The model under review builds one solid part; all positions refer to its coordinate system, in mm. Give positions to 0.01 mm unless a question says otherwise; leave off trailing zeros. Loops run counter-clockwise (first coordinate to the right, second up) from the corner with the lowest first, then second, coordinate; pieces in that order, holes last. Notation, with made-up numbers: M -11.75,15.5 L 7.25,15.5 A16 cw 7.25,46.5 Z; hole C 1,66 d11. An arc over 180 degrees is marked long. Write item = value, one per line. Start each with the question number.
1. We need section A-A on x = 25.5. Give the boundary of the cut face in (y, z).
2. For pin 1 (7 mm diameter, centred on x = 25.5, z = 2, fed in from -Y); pin 2 (1 mm diameter, centred on y = 2, z = 6.5, fed in from -X), all flat-tipped, find the tip position at first contact; note any pin that passes through.
3. We need section B-B on y = 1.35. Give the boundary of the cut face in (x, z) (3 decimals).
4. We need section C-C on z = 7. Give the boundary of the cut face in (x, y).
5. Wall thickness on line 1 along Z through (x, y) = (19, 1.9); line 2 along X through (y, z) = (0.9, 1.5); line 3 along X through (y, z) = (1.9, 0.75): over which ranges is each line inside the solid? List them lowest first. Write a range as from..to.
from build123d import *

# Parameters (mm, degrees)
BOSS_EXTRUDE1_DEPTH = 3
SKETCH2_R           = 1.5
SKETCH2_R_2         = 2.25
SKETCH2_W           = 45.952575141
SKETCH2_H           = 0.01
CUT_EXTRUDE1_DEPTH  = 4


with BuildPart() as part:
    # Sketch1 → Boss-Extrude1 (new body)
    with BuildSketch(Plane(origin=(0, 0, 0), x_dir=(1, 0, 0), z_dir=(0, 1, 0))):
        with BuildLine():
            Line((-37, 4), (37, 4))
            ThreePointArc((37, 4), (39.121320344, 3.121320344), (40, 1))
            Line((40, 1), (40, -5))
            ThreePointArc((40, -5), (39.121320344, -7.121320344), (37, -8))
            Line((37, -8), (-37, -8))
            ThreePointArc((-37, -8), (-39.121320344, -7.121320344), (-40, -5))
            Line((-40, -5), (-40, 1))
            ThreePointArc((-40, 1), (-39.121320344, 3.121320344), (-37, 4))
        make_face()
    extrude(amount=BOSS_EXTRUDE1_DEPTH)

    # Sketch2 → Cut-Extrude1 (cut, through all)
    with BuildSketch(Plane(origin=(0, 3, 0), x_dir=(1, 0, 0), z_dir=(0, 1, 0))):
        with Locations((32, -2)):
            Circle(SKETCH2_R)
        with Locations((25.5, -2)):
            Circle(SKETCH2_R_2)
        with Locations((19, -2)):
            Circle(SKETCH2_R)
        with Locations((-17.02371243, -2)):
            Rectangle(SKETCH2_W, SKETCH2_H)
    extrude(amount=-CUT_EXTRUDE1_DEPTH, mode=Mode.SUBTRACT)


solid = part.part
Final values:
q1.outline = M 0,-4 L 3,-4 L 3,-0.25 L 0,-0.25 Z; M 0,4.25 L 3,4.25 L 3,8 L 0,8 Z
q2.pin_1 = 0
q2.pin_2 = -39.83
q3.outline = M -40,-1 A3 ccw -37,-4 L 37,-4 A3 ccw 40,-1 L 40,5 A3 ccw 37,8 L -37,8 A3 ccw -40,5 L -40,2.005 L 5.953,2.005 L 5.953,1.995 L -40,1.995 Z; hole C 19,2 d3; hole C 25.5,2 d4.5; hole C 32,2 d3
q4.outline = M -39.24,0 L 39.24,0 L 39.24,3 L -39.24,3 Z
q5.line_1 = -4..0.5, 3.5..8
q5.line_2 = -40..17.59, 20.41..23.31, 27.69..30.59, 33.41..40
q5.line_3 = -40..18.17, 19.83..23.63, 27.37..31.17, 32.83..40
